```python
from build123d import *

# Parameters (mm, degrees)
F1_DEPTH = 2


with BuildPart() as f1:
    # F0 (on Top) → F1 (new body)
    with BuildSketch(Plane.XY):
        with BuildLine():
            Line((13.090277, 5.489357), (1.175571, 14.145898))
            ThreePointArc((1.175571, 14.145898), (0, 14.527864), (-1.175571, 14.145898))
            Line((-1.175571, 14.145898), (-13.090277, 5.489357))
            ThreePointArc((-13.090277, 5.489357), (-13.81682, 4.489357), (-13.81682, 3.253289))
            Line((-13.81682, 3.253289), (-11.091217, -5.135255))
            Line((-11.091217, -5.135255), (-8.441377, -5.135255))
            Line((-8.441377, -5.135255), (-8.441377, -7.135255))
            Line((-8.441377, -7.135255), (-10.441377, -7.135255))
            Line((-10.441377, -7.135255), (-9.265807, -10.753289))
            ThreePointArc((-9.265807, -10.753289), (-8.539264, -11.753289), (-7.363694, -12.135255))
            Line((-7.363694, -12.135255), (7.363694, -12.135255))
            ThreePointArc((7.363694, -12.135255), (8.539264, -11.753289), (9.265807, -10.753289))
            Line((9.265807, -10.753289), (10.441377, -7.135255))
            Line((10.441377, -7.135255), (8.441377, -7.135255))
            Line((8.441377, -7.135255), (8.441377, -5.135255))
            Line((8.441377, -5.135255), (11.091217, -5.135255))
            Line((11.091217, -5.135255), (13.81682, 3.253289))
            ThreePointArc((13.81682, 3.253289), (13.81682, 4.489357), (13.090277, 5.489357))
        make_face()
    extrude(amount=F1_DEPTH)


solid = f1.part
```
The listing builds one solid part. Answer for the finished solid, in the listing's coordinates (mm). A direction names the side the tool comes from. Round coordinates to 2 decimals unless told otherwise and drop trailing zeros. Loops run counter-clockwise (first coordinate to the right, second up) from the corner with the lowest first, then second, coordinate; pieces in that order, holes last.
Q1. Which of the six approach directions +Z, -Z, +X, -X, +Y, -Y give full straight-line access (tool end or side, diameter ignored) to faces 1 (the face through (9, -7.135, 1)), 2 (the face through (-8.441, -6, 1)), 3 (the face through (0, 1, 2))?
Q2. Section B-B, the plane z = 1.4 is taken. Determine the outline of the cut face in (x, y), then the cut area to 3 significant figures.
Q3. Section A-A, the plane x = 9.75 is taken. Determine the outline of the cut face in (y, z).
Q4. Section D-D, the plane x = -2.5 is taken. Determine the outline of the cut face in (y, z).
Q5. Find the intervals of material crossed by line 1 (X direction, y = 3.75, z = 0.45); line 2 (X direction, y = -6.5, z = 0.6); line 3 (Y direction, x = 4.75, z = 0.85), in increasing order.
Q6. Section C-C, the plane y = -6.75 is taken. Determine the outline of the cut face in (x, z).
Q7. Given pin 1 Ø8 at (x, y) = (-10.5, 6.5) entering from -Z; pin 2 Ø1 at (x, z) = (9.5, 1) entering from +Y; pin 3 Ø1 at (x, z) = (-5, 0) entering from +Y; pin 4 Ø0.6 at (y, z) = (-5.5, 0.5) entering from -X, each flat-ended and moving along its own axis, determine where each tip first touches the part or whether it passes through.
Completed:
1. face 1: +Z, -Z, +X
1. face 2: +Z, -Z, -X
1. face 3: +Z, +X, -X, +Y, -Y
2. outline: (-13.82, 3.25) - (-11.09, -5.14) - (-8.44, -5.14) - (-8.44, -7.14) - (-10.44, -7.14) - (-9.27, -10.75) arc R2 ccw to (-7.36, -12.14) - (7.36, -12.14) arc R2 ccw to (9.27, -10.75) - (10.44, -7.14) - (8.44, -7.14) - (8.44, -5.14) - (11.09, -5.14) - (13.82, 3.25) arc R2 ccw to (13.09, 5.49) - (1.18, 14.15) arc R2 ccw to (-1.18, 14.15) - (-13.09, 5.49) arc R2 ccw to start
2. area: 524 mm2
3. outline: (-9.26, 0) - (-7.14, 0) - (-7.14, 2) - (-9.26, 2) - close; (-5.14, 0) - (7.92, 0) - (7.92, 2) - (-5.14, 2) - close
4. outline: (-12.14, 0) - (13.18, 0) - (13.18, 2) - (-12.14, 2) - close
5. line 1: x = -13.91 to 13.91
5. line 2: x = -8.44 to 8.44
5. line 3: y = -12.14 to 11.55
6. outline: (-8.44, 0) - (8.44, 0) - (8.44, 2) - (-8.44, 2) - close
7. pin 1: stops at z = 0
7. pin 2: stops at y = 8.46
7. pin 3: stops at y = 11.73
7. pin 4: stops at x = -8.44
